Input: part model. Units: mm. Frame: model coordinates. A direction names the side the tool comes from. Coordinates: 2 decimals unless noted, no trailing zeros. Order: outer loops, then holes, each group sorted by start corner. A loop starts at its lowest first (then second) coordinate and runs counter-clockwise, first axis right, second up. Notation, with made-up numbers: (-27, -0.75) -> (15, -0.75) arc R8 ccw to (15, 11.25) -> close; hole circle Ø2 at (32.5, 31.5). An arc over 180 degrees is marked (long way). One line per question, with ' | ' between items.
```python
from build123d import *

# Parameters (mm, degrees)
SKETCH1_R                      = 7.9375
BOSS_EXTRUDE1_DEPTH            = 76.2
M6X1_0_TAPPED_HOLE1_D          = 5
M6X1_0_TAPPED_HOLE1_DEPTH      = 29.9999908
M6X1_0_TAPPED_HOLE1_TIP        = 1.502151548
F_10_0_10_DIAMETER_HOLE2_D     = 10
F_10_0_10_DIAMETER_HOLE2_DEPTH = 13.9999974
F_10_0_10_DIAMETER_HOLE2_TIP   = 3.004303095
F_8_32_TAPPED_HOLE1_D          = 3.4544
SKETCH15_R                     = 7.9375
SKETCH15_R_2                   = 6.35
CUT_EXTRUDE2_DEPTH             = 57.15


with BuildPart() as part:
    # Sketch1 → Boss-Extrude1 (new body)
    with BuildSketch(Plane(origin=(0, 0, 0), x_dir=(1, 0, 0), z_dir=(0, 1, 0))):
        Circle(SKETCH1_R)
    extrude(amount=BOSS_EXTRUDE1_DEPTH)

    # M6x1.0 Tapped Hole1
    with Locations(Plane(origin=(0, 0, 0), x_dir=(-1, 0, 0), z_dir=(0, -1, 0))):
        with Locations((0, 0)):
            Hole(M6X1_0_TAPPED_HOLE1_D / 2, depth=M6X1_0_TAPPED_HOLE1_DEPTH)
            with Locations((0, 0, -(M6X1_0_TAPPED_HOLE1_DEPTH + M6X1_0_TAPPED_HOLE1_TIP / 2))):  # 118° drill point
                Cone(0, M6X1_0_TAPPED_HOLE1_D / 2, M6X1_0_TAPPED_HOLE1_TIP, mode=Mode.SUBTRACT)

    # Ø10.0 (10) Diameter Hole2
    with Locations(Plane(origin=(0, 0, 0), x_dir=(-1, 0, 0), z_dir=(0, -1, 0))):
        with Locations((0, 0)):
            Hole(F_10_0_10_DIAMETER_HOLE2_D / 2, depth=F_10_0_10_DIAMETER_HOLE2_DEPTH)
            with Locations((0, 0, -(F_10_0_10_DIAMETER_HOLE2_DEPTH + F_10_0_10_DIAMETER_HOLE2_TIP / 2))):  # 118° drill point
                Cone(0, F_10_0_10_DIAMETER_HOLE2_D / 2, F_10_0_10_DIAMETER_HOLE2_TIP, mode=Mode.SUBTRACT)

    # #8-32 Tapped Hole1 (through all)
    with Locations(Plane.XY.offset(7.9375)):
        with Locations((0, 6.35)):
            Hole(F_8_32_TAPPED_HOLE1_D / 2)

    # Sketch15 → Cut-Extrude2 (cut)
    with BuildSketch(Plane(origin=(0, 76.2, 0), x_dir=(1, 0, 0), z_dir=(0, 1, 0))):
        Circle(SKETCH15_R)
        Circle(SKETCH15_R_2, mode=Mode.SUBTRACT)
    extrude(amount=-CUT_EXTRUDE2_DEPTH, mode=Mode.SUBTRACT)


solid = part.part
```
1. Cut plane B-B, the plane y = 20. Return loops of the section in (x, z), and give its area (3 significant figures).
Recorded:
outline: circle Ø12.7 at (0, 0); hole circle Ø5 at (0, 0) | area: 107 mm^2
2. Ray query, line 1 (Z direction, x = 0, y = 20); line 2 (Y direction, x = 0, z = -5.9); line 3 (Z direction, x = 0, y = 3.5). Return the intervals inside material, ascending. Write a range as [from, to].
Recorded:
line 1: z = [-6.35, -2.5], [2.5, 6.35] | line 2: y = [0, 4.62], [8.08, 76.2] | line 3: z = [-7.94, -5], [5, 7.94]
3. Mould query, pull axis Y, two halves, no side actions, for faces 3 (the face through (1.726, 6.426, 6.295)), 4 (the face through (0, 19.05, -7)), 5 (the face through (-1.38, 48.03, 6.2)). Classes: released by +Y, released by -Y, zero draft, split by the parting line, or undercut.
Recorded:
face 3: undercut | face 4: released by +Y | face 5: zero draft
4. Access query for faces 1 (the face through (4.77, 7.1, -1.5)), 2 (the face through (-1.72, 9.39, 7.75)). Directions: +Z, -Z, +X, -X, +Y, -Y. A direction counts if a zero-diameter tool reaches every point of the face in a straight line with its end or side. Return the directions, or none.
Recorded:
face 1: -Y | face 2: +Y, -Y
5. Pin query (flat end, axial travel): pin 1 Ø6 at (y, z) = (62, 1) entering from +X; pin 2 Ø8 at (x, y) = (-1, 56) entering from +Z; pin 3 Ø4 at (x, y) = (6, 11.5) entering from +Z; pin 4 Ø3 at (x, y) = (0, 6.35) entering from -Z. Return the tip coordinate at first contact, or that it passes through.
Recorded:
pin 1: stops at x = 6.35 | pin 2: stops at z = 6.35 | pin 3: stops at z = 6.86 | pin 4: passes through
6. Cut plane C-C, the plane y = 47. Return loops of the section in (x, z), and give its area (3 significant figures).
Recorded:
outline: circle Ø12.7 at (0, 0) | area: 127 mm^2
7. Cut plane A-A, the plane y = 6.35. Return loops of the section in (x, z) (1 decimal), and give its area (3 significant figures).
Recorded:
outline: (-1.7, -7.7) -> (-1.7, -4.7) arc R5 cw to (-1.7, 4.7) -> (-1.7, 7.7) arc R7.9 ccw to start; (1.7, -7.7) arc R7.9 ccw to (1.7, 7.7) -> (1.7, 4.7) arc R5 cw to (1.7, -4.7) -> close | area: 98.8 mm^2
